from build123d import *

# Parameters (mm, degrees)
BOSS_EXTRUDE1_DEPTH   = 28
BOSS_EXTRUDE1_2_DEPTH = 28
SKETCH1_4_R           = 36
BOSS_EXTRUDE2_DEPTH   = 55
SKETCH1_5_R           = 13
CUT_EXTRUDE1_DEPTH    = 95.21915941
CUT_EXTRUDE2_START    = -10
CUT_EXTRUDE2_DEPTH    = 10
SKETCH2_3_W           = 26
SKETCH2_3_H           = 91.506160118
CUT_EXTRUDE3_DEPTH    = 24
SKETCH3_W             = 36
SKETCH3_H             = 32
CUT_EXTRUDE4_DEPTH    = 20


with BuildPart() as part:
    # Sketch1 → Boss-Extrude1 (new body)
    with BuildSketch(Plane(origin=(0, 0, 0), x_dir=(1, 0, 0), z_dir=(0, 1, 0))):
        with BuildLine():
            Line((-67.5, 28), (-67.5, -28))
            Line((-67.5, -28), (-22.627416998, -28))
            ThreePointArc((-22.627416998, -28), (-36, 0), (-22.627416998, 28))
            Line((-22.627416998, 28), (-67.5, 28))
        make_face()
    extrude(amount=BOSS_EXTRUDE1_DEPTH)



with BuildPart() as body_2:
    # Sketch1 → Boss-Extrude1 2 (new body)
    with BuildSketch(Plane(origin=(0, 0, 0), x_dir=(1, 0, 0), z_dir=(0, 1, 0))):
        with BuildLine():
            ThreePointArc((36, 0), (32.485281374, -15.514718626), (22.627416998, -28))
            Line((22.627416998, -28), (67.5, -28))
            Line((67.5, -28), (67.5, 28))
            Line((67.5, 28), (22.627416998, 28))
            ThreePointArc((22.627416998, 28), (32.485281374, 15.514718626), (36, 0))
        make_face()
    extrude(amount=BOSS_EXTRUDE1_2_DEPTH)


with BuildPart() as part_1:
    add(part.part)

    add(body_2.part)  # Boss-Extrude2 merges body 2
    # Sketch1_4 → Boss-Extrude2 (add)
    with BuildSketch(Plane(origin=(0, 0, 0), x_dir=(1, 0, 0), z_dir=(0, 1, 0))):
        with Locations(Location((0, 0, 0), (0, 0, 51.057558731))):
            Circle(SKETCH1_4_R)
    extrude(amount=BOSS_EXTRUDE2_DEPTH)

    # Sketch1_5 → Cut-Extrude1 (cut, through all)
    with BuildSketch(Plane(origin=(0, 0, 0), x_dir=(1, 0, 0), z_dir=(0, 1, 0))):
        with Locations(Location((0, 0, 0), (0, 0, 270))):
            Circle(SKETCH1_5_R)
    extrude(amount=CUT_EXTRUDE1_DEPTH, mode=Mode.SUBTRACT)

    # Sketch2 → Cut-Extrude2 (cut)
    with BuildSketch(Plane(origin=(0, 55, 0), x_dir=(1, 0, 0), z_dir=(0, 1, 0)).offset(CUT_EXTRUDE2_START)):
        with BuildLine():
            Line((13, 0), (13, -21.354156504))
            ThreePointArc((13, -21.354156504), (21.794494718, -12.247448714), (25, 0))
            ThreePointArc((25, 0), (21.794494718, 12.247448714), (13, 21.354156504))
            Line((13, 21.354156504), (13, 0))
        make_face()
        with BuildLine():
            Line((-13, -1.1e-08), (-13, -21.354156504))
            ThreePointArc((-13, -21.354156504), (0, -25), (13, -21.354156504))
            Line((13, -21.354156504), (13, 0))
            ThreePointArc((13, 0), (6e-09, -13), (-13, -1.1e-08))
        make_face()
        with BuildLine():
            Line((-13, 21.354156504), (-13, -1.1e-08))
            ThreePointArc((-13, -1.1e-08), (-6e-09, 13), (13, 0))
            Line((13, 0), (13, 21.354156504))
            ThreePointArc((13, 21.354156504), (0, 25), (-13, 21.354156504))
        make_face()
        with BuildLine():
            ThreePointArc((-13, 21.354156504), (-25, 0), (-13, -21.354156504))
            Line((-13, -21.354156504), (-13, -1.1e-08))
            Line((-13, -1.1e-08), (-13, 21.354156504))
        make_face()
    extrude(amount=CUT_EXTRUDE2_DEPTH, mode=Mode.SUBTRACT)

    # Sketch2_3 → Cut-Extrude3 (cut)
    with BuildSketch(Plane(origin=(0, 55, 0), x_dir=(1, 0, 0), z_dir=(0, 1, 0))):
        Rectangle(SKETCH2_3_W, SKETCH2_3_H)
    extrude(amount=-CUT_EXTRUDE3_DEPTH, mode=Mode.SUBTRACT)

    # Sketch3 → Cut-Extrude4 (cut)
    with BuildSketch(Plane(origin=(0, 28, 0), x_dir=(1, 0, 0), z_dir=(0, 1, 0))):
        with Locations((67.5, 0)):
            Rectangle(SKETCH3_W, SKETCH3_H)
        with Locations((-67.5, 0)):
            Rectangle(SKETCH3_W, SKETCH3_H)
    extrude(amount=-CUT_EXTRUDE4_DEPTH, mode=Mode.SUBTRACT)


solid = part_1.part
Can you work these out from the model? Positions are in its coordinate system, mm. A direction names the side the tool comes from. Give positions to 0.01 mm unless a question says otherwise; leave off trailing zeros. Loops run counter-clockwise (first coordinate to the right, second up) from the corner with the lowest first, then second, coordinate; pieces in that order, holes last. Notation, with made-up numbers: (25.5, 82) - (41.5, 82) arc R8 ccw to (41.5, 90) - close; hole circle Ø10 at (0.5, 46.5). An arc over 180 degrees is marked (long way). Return JSON: item names as keys, results as strings.
1. If I drill on line 1 (Z direction, x = -60, y = 26); line 2 (Z direction, x = 0, y = 8); line 3 (Z direction, x = -44, y = 23), over which ranges is the centre line in solid material (lowest first)?
Output values:
{"line 1": "z = -28 to -16, 16 to 28", "line 2": "z = -36 to -13, 13 to 36", "line 3": "z = -28 to 28"}
2. I want a section at D-D on y = 46.5. Please give me the cut outline in (x, z), and give its area (3 significant figures).
Output values:
{"outline": "(-13, -33.57) - (-13, -21.35) arc R25 cw to (-13, 21.35) - (-13, 33.57) arc R36 ccw to start; (13, -33.57) arc R36 ccw to (13, 33.57) - (13, 21.35) arc R25 cw to (13, -21.35) - close", "area": "1,520 mm²"}
3. I want a section at C-C on z = -4.5. Please give me the cut outline in (x, y).
Output values:
{"outline": "(-67.5, 0) - (-12.2, 0) - (-12.2, 31) - (-13, 31) - (-13, 45) - (-24.59, 45) - (-24.59, 55) - (-35.72, 55) - (-35.72, 28) - (-49.5, 28) - (-49.5, 8) - (-67.5, 8) - close; (12.2, 0) - (67.5, 0) - (67.5, 8) - (49.5, 8) - (49.5, 28) - (35.72, 28) - (35.72, 55) - (24.59, 55) - (24.59, 45) - (13, 45) - (13, 31) - (12.2, 31) - close"}
4. We'd pull the mould along X, two halves only. Please class faces 5 (the face through (0, 31, -22)), 6 (the face through (58, 8, 0)), 7 (the face through (-67.5, 7.6, -0.4)), 8 (the face through (0, 31, 22)): +X half, -X half, draft (parallel to the pull), parting line (faces both ways), or undercut.
Output values:
{"face 5": "undercut", "face 6": "draft", "face 7": "-X half", "face 8": "undercut"}
5. I'm going to push flat-ended pins straight in: pin 1 Ø6 at (x, z) = (-16.5, 3) entering from +Y; pin 2 Ø9 at (x, y) = (54.5, 15) entering from -Z; pin 3 Ø8 at (x, z) = (-4, 13.5) entering from +Y. Where does each tip first touch, or does it pass through?
Output values:
{"pin 1": "stops at y = 45", "pin 2": "stops at z = -28", "pin 3": "stops at y = 31"}
6. I want a section at A-A on y = 12. Please give me the cut outline in (x, z).
Output values:
{"outline": "(-67.5, -28) - (-22.63, -28) arc R36 ccw to (22.63, -28) - (67.5, -28) - (67.5, -16) - (49.5, -16) - (49.5, 16) - (67.5, 16) - (67.5, 28) - (22.63, 28) arc R36 ccw to (-22.63, 28) - (-67.5, 28) - (-67.5, 16) - (-49.5, 16) - (-49.5, -16) - (-67.5, -16) - close; hole circle Ø26 at (0, 0)"}
7. I want a section at B-B on x = 0. Please give me the cut outline in (y, z).
Output values:
{"outline": "(0, -36) - (31, -36) - (31, -13) - (0, -13) - close; (0, 13) - (31, 13) - (31, 36) - (0, 36) - close"}
8. For faces 1 (the face through (49.5, 18, 0)), 2 (the face through (-45, 14, -28)), 3 (the face through (45, 14, 28)), 4 (the face through (-59, 18, 16)), which set-ups out of +Z, -Z, +X, -X, +Y, -Y let a thin tool reach every point of the face, with its end or its side?
Output values:
{"face 1": "+X, +Y", "face 2": "-Z, -X, +Y, -Y", "face 3": "+Z, +X, +Y, -Y", "face 4": "-X, +Y"}
